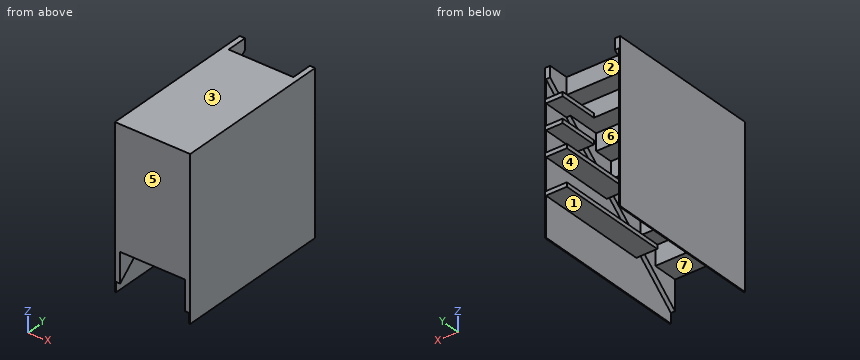
```python
from build123d import *

# Parameters (mm, degrees)
F0_W          = 914.4
F0_H          = 1930.4
F1_DEPTH      = 1930.4
F3_DEPTH      = 393.7
F3_DEPTH_BACK = 393.7
F5_DEPTH      = 444.5
F5_DEPTH_BACK = 444.5
F6_W          = 254
F6_H          = 50.8
F6_W_2        = 203.2
F7_DEPTH      = 482.6
F8_W          = 254
F8_H          = 50.8
F9_DEPTH      = 1397
F10_W         = 254
F10_H         = 50.8
F11_DEPTH     = 939.8


with BuildPart() as f1:
    # F0 (on Front) → F1 (new body)
    with BuildSketch(Plane.XZ):
        Rectangle(F0_W, F0_H)
    extrude(amount=F1_DEPTH)

    # F2 (on Right) → F3 (cut, two sides)
    with BuildSketch(Plane.YZ) as f3_sk:
        Polygon((81.8748995662, 971.9918370247), (-254, 965.2), (-254, 762), (-482.6, 762), (-482.6, 558.8), (-711.2, 558.8), (-711.2, 355.6), (-939.8, 355.6), (-939.8, 152.4), (-1168.4, 152.4), (-1168.4, -50.8), (-1397, -50.8), (-1397, -254), (-1625.6, -254), (-1625.6, -485.139220953), (-1930.4, -485.139220953), (-1930.4, -969.014108181), (215.3691798449, -969.014108181), align=None)
    extrude(amount=-F3_DEPTH, mode=Mode.SUBTRACT)
    extrude(f3_sk.sketch, amount=F3_DEPTH_BACK, mode=Mode.SUBTRACT)

    # F4 (on Right) → F5 (cut, two sides)
    with BuildSketch(Plane.YZ) as f5_sk:
        Polygon((233.0105304718, -1000.3662109375), (0, 832.7655792236), (-1940.5599832535, -853.7156581879), (-2034.8353385925, -1000.3662109375), align=None)
    extrude(amount=-F5_DEPTH, mode=Mode.SUBTRACT)
    extrude(f5_sk.sketch, amount=F5_DEPTH_BACK, mode=Mode.SUBTRACT)

    # F6 (on face) → F7 (join, through all)
    with BuildSketch(Plane(origin=(0, 0, 0), x_dir=(-1, 0, 0), z_dir=(0, 1, 0))):
        with Locations((-317.5, -463.55)):
            Rectangle(F6_W, F6_H)
        with Locations((-317.5, -25.4)):
            Rectangle(F6_W, F6_H)
        with Locations((-342.9, 279.4)):
            Rectangle(F6_W_2, F6_H)
        with Locations((-342.9, 584.2)):
            Rectangle(F6_W_2, F6_H)
    extrude(amount=-F7_DEPTH)

    # F8 (on face) → F9 (join, through all)
    with BuildSketch(Plane(origin=(0, 0, 0), x_dir=(-1, 0, 0), z_dir=(0, 1, 0))):
        with Locations((-317.5, -463.55)):
            Rectangle(F8_W, F8_H)
    extrude(amount=-F9_DEPTH)

    # F10 (on face) → F11 (join, through all)
    with BuildSketch(Plane(origin=(0, 0, 0), x_dir=(-1, 0, 0), z_dir=(0, 1, 0))):
        with Locations((-317.5, -25.4)):
            Rectangle(F10_W, F10_H)
    extrude(amount=-F11_DEPTH)


solid = f1.part
```
The model under review builds one solid part; all positions refer to its coordinate system, in mm. Face numbers are marked on the shaded views. A direction names the side the tool comes from. Coordinates: 2 decimals unless noted, no trailing zeros. Write each loop counter-clockwise with the first axis right and the second up, starting at its lowest first coordinate (ties: lowest second). Pieces come first, ordered by that corner, then holes.
1) To check wall thickness, follow probe 1 along Z at (x, y) = (375, -200); probe 2 along Z at (x, y) = (206, -629.5); probe 3 along X at (y, z) = (-331, 219). State the ranges of each line that lie inside material, in increasing order.
2) The part is to be moulded in two halves that separate along Z. For the marked faces 1, 2, 3 and 4, say which applies: pulls with the +Z half, pulls with the -Z half, needs draft (parallel to the pull), parting line crosses it, or undercut.
3) Machinability: for the marked faces 5, 6 and 7, which of the approach directions +Z, -Z, +X, -X, +Y, -Y give a long, thin tool a straight path to every point of the face, cutting with its end or side? Answer none if there is none.
4) We need section C-C on z = 79. State the section outline as (x, y) points, then the cut area to 3 significant figures.
5) We need section A-A on y = -190.5. State the section outline as (x, z) points, then the cut area to 3 significant figures.
6) We need section B-B on x = 14. State the section outline as (y, z) points, then the cut area to 3 significant figures.
7) Clearance check with flat-ended pins moving along their axes: pin 1 Ø10 at (x, z) = (-201, 170.5) entering from +Y; pin 2 Ø1 at (x, y) = (151, -330) entering from -Z. State where each tip first meets the part, or that it passes through.
8) We need section D-D on y = -1467. State the section outline as (x, z) points, then the cut area to 3 significant figures.
Answer list:
1. probe 1: z = -488.95 to -438.15, -50.8 to 0, 254 to 304.8, 558.8 to 609.6
1. probe 2: z = -488.95 to -438.15, -50.8 to 0, 558.8 to 965.2
1. probe 3: x = -457.2 to -444.5, 444.5 to 457.2
2. face 1: pulls with the -Z half
2. face 2: needs draft
2. face 3: pulls with the +Z half
2. face 4: undercut
3. face 5: +Z, -Z, +X, -X, -Y
3. face 6: +Y
3. face 7: -Z, -Y
4. outline: (-457.2, -1930.4) - (457.2, -1930.4) - (457.2, 0) - (444.5, 0) - (444.5, -867.32) - (393.7, -867.32) - (393.7, -1168.4) - (-393.7, -1168.4) - (-393.7, -867.32) - (-444.5, -867.32) - (-444.5, 0) - (-457.2, 0) - close
4. area: 757,000 mm2
5. outline: (-457.2, -965.2) - (-444.5, -965.2) - (-444.5, 667.21) - (-393.7, 667.21) - (-393.7, 965.2) - (-457.2, 965.2) - close; (190.5, -488.95) - (444.5, -488.95) - (444.5, -965.2) - (457.2, -965.2) - (457.2, 965.2) - (393.7, 965.2) - (393.7, 667.21) - (444.5, 667.21) - (444.5, 609.6) - (241.3, 609.6) - (241.3, 558.8) - (444.5, 558.8) - (444.5, 304.8) - (241.3, 304.8) - (241.3, 254) - (444.5, 254) - (444.5, 0) - (190.5, 0) - (190.5, -50.8) - (444.5, -50.8) - (444.5, -438.15) - (190.5, -438.15) - close
5. area: 126,000 mm2
6. outline: (-1930.4, -485.14) - (-1625.6, -485.14) - (-1625.6, -254) - (-1397, -254) - (-1397, -50.8) - (-1168.4, -50.8) - (-1168.4, 152.4) - (-939.8, 152.4) - (-939.8, 355.6) - (-711.2, 355.6) - (-711.2, 558.8) - (-482.6, 558.8) - (-482.6, 762) - (-254, 762) - (-254, 965.2) - (-1930.4, 965.2) - close
6. area: 1,420,000 mm2
7. pin 1: stops at y = -939.8
7. pin 2: stops at z = 762
8. outline: (-457.2, -965.2) - (-444.5, -965.2) - (-444.5, -442.16) - (-393.7, -442.16) - (-393.7, -254) - (393.7, -254) - (393.7, -442.16) - (444.5, -442.16) - (444.5, -965.2) - (457.2, -965.2) - (457.2, 965.2) - (-457.2, 965.2) - close
8. area: 1,150,000 mm2
